Read the model definition and answer for the solid it produces. Units are mm, in the model's axes. Face numbers are marked on the shaded views. A direction names the side the tool comes from. Round coordinates to 2 decimals unless told otherwise and drop trailing zeros. Order: outer loops, then holes, each group sorted by start corner. A loop starts at its lowest first (then second) coordinate and runs counter-clockwise, first axis right, second up. Notation, with made-up numbers: (-1.75, 58.5) - (37.25, 58.5) arc R23 ccw to (37.25, 89.5) - close; hole circle Ø9 at (68, -29.75). An arc over 180 degrees is marked (long way). Put each result on its own line as item: value. Start each with the question number.
Q1. Section B-B on y = 8 is taken. Give the vertices of the cut face in (x, z) (3 decimals).
Q2. Section C-C on x = 17.5 is taken. Give the vertices of the cut face in (y, z) (3 decimals).
Q3. Find the intervals of material crossed by line 1 along Z through (x, y) = (-25.5, 7.5); line 2 along X through (y, z) = (-14.5, 19.5) (3 decimals); line 3 along Y through (x, z) = (-12.5, 12.5), in increasing order. Write a range as from..to.
Q4. For a pull along Z with two mould halves and no side action, classify the marked faces 1, 2, 3 and 4 as pulls with the +Z half, pulls with the -Z half, needs draft (parallel to the pull), parting line crosses it, or undercut.
Q5. Each of these flat-tipped pins is pushed along its axis until it touches: pin 1 Ø0.6 at (x, y) = (-47.5, 8) entering from -Z; pin 2 Ø0.6 at (x, y) = (-47, 8) entering from +Z; pin 3 Ø6 at (x, z) = (-24, 40.5) entering from -Y. Where does it stop, or does it pass through?
Q6. Section A-A on z = 6 is taken. Give the vertices of the cut face in (x, y) (3 decimals).
Q7. Section D-D on y = -12 is taken. Give the vertices of the cut face in (x, z) (3 decimals).
Q8. Which of the six approach directions +Z, -Z, +X, -X, +Y, -Y give full straight-line access (tool end or side, diameter ignored) to the marked faces 5 and 6?
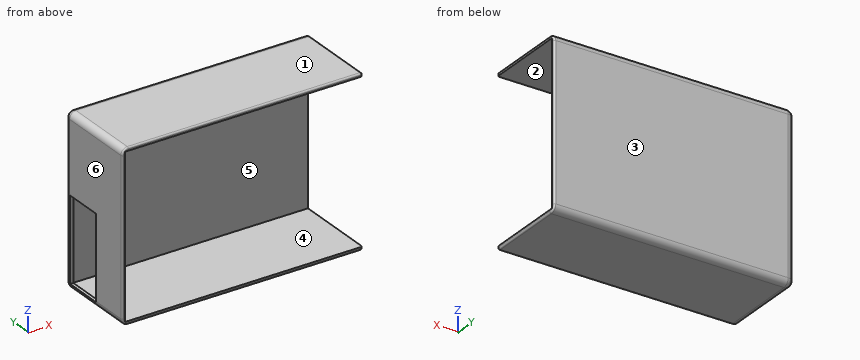
Autodesk Inventor part; units mm, degrees
ref_plane "YZ Plane" through (0, 0, 0) normal (1, 0, 0) x (0, 1, 0)
ref_plane "XZ Plane" through (0, 0, 0) normal (0, 1, 0) x (-1, 0, 0)
ref_plane "XY Plane" through (0, 0, 0) normal (0, 0, 1) x (1, 0, 0)
sketch "Sketch1" plane through (0, 0, 0) normal (0, 0, 1) x (1, 0, 0)
  line L0 (-47.625, -16.6751) -> (47.625, -16.6751)
  line L1 (47.625, -16.6751) -> (47.625, 16.6751)
  line L2 (47.625, 16.6751) -> (-47.625, 16.6751)
  line L3 (-47.625, 16.6751) -> (-47.625, -16.6751)
  line L4 (-47.625, -16.6751) -> (47.625, 16.6751) construction
  line L5 (47.625, -16.6751) -> (-47.625, 16.6751) construction
  point P0 (0, 0)
  dimension "d0" = 95.25
  dimension "d1" = 33.3502
extrude "Extrusion1" add sketch "Sketch1" along normal blind 66.04
shell "Shell1" thickness 1.27 removed faces 2 at (47.625, -5.5584, 44.0267) at (-15.875, -16.6751, 44.0267)
sketch "Sketch2" plane through (-46.355, -16.6751, 1.27) normal (1, 0, 0) x (0, 0, -1)
  line L0 (0, 32.0802) -> (0, 0)
  line L1 (0, 0) -> (-63.5, 0)
  line L2 (-33.9598, 15.2908) -> (-0.9398, 15.2908)
  line L3 (-0.9398, 15.2908) -> (-0.9398, 30.5308)
  line L4 (-0.9398, 30.5308) -> (-33.9598, 30.5308)
  line L5 (-33.9598, 30.5308) -> (-33.9598, 15.2908)
  line L6 (-33.9598, 15.2908) -> (-0.9398, 30.5308) construction
  line L7 (-0.9398, 15.2908) -> (-33.9598, 30.5308) construction
  point P0 (1.27, 16.6751)
  point P1 (-17.4498, 22.9108)
  dimension "d5" = 17.4498
  dimension "d6" = 22.9108
  dimension "d13" = 33.02
  dimension "d14" = 15.24
extrude "Extrusion2" cut sketch "Sketch2" against normal up to surface (1.27 mm away)
fillet "Fillet1" radius 2.54 5 edges at (0, 16.6751, 66.04) (-47.625, 16.6751, 33.02) (0, 16.6751, 0) (-47.625, 0, 0) (-47.625, 0, 66.04)
fillet "Fillet2" radius 0.635 5 edges at (47.625, -1.27, 0) (47.625, 15.9312, 0.7439) (47.625, 16.6751, 33.02) (47.625, 15.9312, 65.2961) (47.625, -1.27, 66.04)
fillet "Fillet3" radius 0.635 9 edges at (47.439, -16.6751, 65.854) (47.625, -16.6751, 65.0875) (-46.8811, -16.6751, 65.2961) (-47.625, -16.6751, 33.02) (-46.8811, -16.6751, 0.7439) (0.9525, -16.6751, 0) (47.439, -16.6751, 0.186) (47.625, -16.6751, 0.9525) (0.9525, -16.6751, 66.04)
properties part number "SPO2_cover"
Findings:
1. outline: (-47.625, 35.23) - (-46.355, 35.23) - (-46.355, 64.77) - (47.625, 64.77) - (47.625, 65.405) arc R0.635 ccw to (46.99, 66.04) - (-45.085, 66.04) arc R2.54 ccw to (-47.625, 63.5) - close; (-47.603, 2.21) arc R2.54 ccw to (-45.085, 0) - (46.99, 0) arc R0.635 ccw to (47.625, 0.635) - (47.625, 1.27) - (-46.355, 1.27) - (-46.355, 2.21) - close
2. outline: (-16.675, 0.635) arc R0.635 ccw to (-16.04, 0) - (14.135, 0) arc R2.54 ccw to (16.675, 2.54) - (16.675, 63.5) arc R2.54 ccw to (14.135, 66.04) - (-16.04, 66.04) arc R0.635 ccw to (-16.675, 65.405) - (-16.675, 64.77) - (15.405, 64.77) - (15.405, 1.27) - (-16.675, 1.27) - close
3. line 1: 0..1.27, 64.77..66.04
3. line 2: -47.625..-46.355
3. line 3: 15.41..16.68
4. face 1: pulls with the +Z half
4. face 2: undercut
4. face 3: needs draft
4. face 4: undercut
5. pin 1: z = 1.13
5. pin 2: z = 65.46
5. pin 3: y = 15.41
6. outline: (-47.625, -16.04) arc R0.635 ccw to (-46.99, -16.675) - (-46.355, -16.675) - (-46.355, -1.384) - (-47.625, -1.384) - close; (-47.625, 13.856) - (-46.355, 13.856) - (-46.355, 15.405) - (47.625, 15.405) - (47.625, 16.04) arc R0.635 ccw to (46.99, 16.675) - (-45.085, 16.675) arc R2.54 ccw to (-47.625, 14.135) - close
7. outline: (-47.625, 2.54) arc R2.54 ccw to (-45.085, 0) - (46.99, 0) arc R0.635 ccw to (47.625, 0.635) - (47.625, 1.27) - (-46.355, 1.27) - (-46.355, 64.77) - (47.625, 64.77) - (47.625, 65.405) arc R0.635 ccw to (46.99, 66.04) - (-45.085, 66.04) arc R2.54 ccw to (-47.625, 63.5) - close
8. face 5: +X, -Y
8. face 6: +Z, -Z, -X, +Y, -Y
